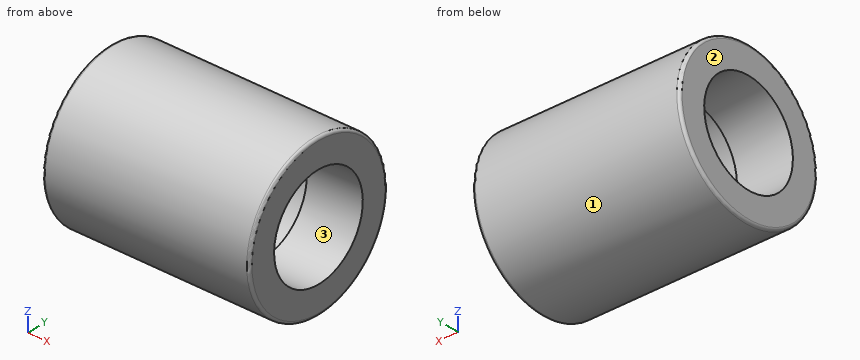
from build123d import *

# Parameters (mm, degrees)
F2_R = 0.5


with BuildPart() as f1:
    # F0 (on Front) → F1 (revolve)
    with BuildSketch(Plane.XZ):
        with BuildLine():
            Line((34.340206, 14), (-2.659794, 14))
            Line((-2.659794, 14), (-2.659794, 9))
            Line((-2.659794, 9), (7.340206, 9))
            Line((7.340206, 9), (7.340206, 10))
            ThreePointArc((7.340206, 10), (7.633099, 10.707107), (8.340206, 11))
            Line((8.340206, 11), (23.340206, 11))
            ThreePointArc((23.340206, 11), (24.047313, 10.707107), (24.340206, 10))
            Line((24.340206, 10), (24.340206, 9))
            Line((24.340206, 9), (34.340206, 9))
            Line((34.340206, 9), (34.340206, 14))
        make_face()
    revolve(axis=Axis((-0.122449, 0, 0), (1, 0, 0)))

    # F2
    f2_edges = [f1.edges().sort_by_distance(p)[0] for p in [
        (-2.659794, 0, -14),
        (34.340206, 0, -14),
    ]]
    fillet(f2_edges, radius=F2_R)


solid = f1.part
Model file for the job. Use its own axes, mm. Face numbers are marked on the shaded views. Round coordinates to 2 decimals unless told otherwise and drop trailing zeros. Order: outer loops, then holes, each group sorted by start corner. A loop starts at its lowest first (then second) coordinate and runs counter-clockwise, first axis right, second up.
(1) Pull direction Z, two halves, no side cores. Call the marked faces 1, 2 and 3: released by +Z, released by -Z, zero draft, split by the parting line, or undercut.
(2) Pin check, flat tips, straight feed: pin 1 (4 mm diameter, centred on x = 2, z = 10.5, fed in from +Y); pin 2 (4 mm diameter, centred on x = 24, z = 9, fed in from +Y); pin 3 (6 mm diameter, centred on x = 2.5, y = -6.5, fed in from -Z). Stop position of each tip, or through.
(3) Band-saw the part on C-C (x = 19). List the corners of the cut face in (y, z).
(4) Band-saw the part on A-A (y = 0). List the corners of the cut face in (x, z).
(5) Band-saw the part on D-D (x = 32). List the corners of the cut face in (y, z), then the cut area to 3 significant figures.
(6) Drill centre lines: line 1 (Y direction, x = 3.5, z = 0); line 2 (X direction, y = -8.75, z = 4); line 3 (Z direction, x = 13.5, y = 0). Where is each one in solid material? Low to high.
Verdict:
1. face 1: split by the parting line
1. face 2: zero draft
1. face 3: undercut
2. pin 1: stops at y = 11.12
2. pin 2: stops at y = 12.12
2. pin 3: stops at z = -13.56
3. outline: circle Ø28 at (0, 0); hole circle Ø22 at (0, 0)
4. outline: (-2.66, -13.5) arc R0.5 ccw to (-2.16, -14) - (33.84, -14) arc R0.5 ccw to (34.34, -13.5) - (34.34, -9) - (24.34, -9) - (24.34, -10) arc R1 cw to (23.34, -11) - (8.34, -11) arc R1 cw to (7.34, -10) - (7.34, -9) - (-2.66, -9) - close; (-2.66, 9) - (7.34, 9) - (7.34, 10) arc R1 cw to (8.34, 11) - (23.34, 11) arc R1 cw to (24.34, 10) - (24.34, 9) - (34.34, 9) - (34.34, 13.5) arc R0.5 ccw to (33.84, 14) - (-2.16, 14) arc R0.5 ccw to (-2.66, 13.5) - close
5. outline: circle Ø28 at (0, 0); hole circle Ø18 at (0, 0)
5. area: 361 mm2
6. line 1: y = -14 to -9, 9 to 14
6. line 2: x = -2.66 to 7.34, 24.34 to 34.34
6. line 3: z = -14 to -11, 11 to 14
